CAD build for the part. Positions are in the model's coordinates, mm. A direction names the side the tool comes from. Coordinates: 2 decimals unless noted, no trailing zeros. Order: outer loops, then holes, each group sorted by start corner. A loop starts at its lowest first (then second) coordinate and runs counter-clockwise, first axis right, second up. Notation, with made-up numbers: (54, 72.5) - (77, 72.5) arc R23 cw to (77, 83.5) - close; hole circle Ø2 at (-8, 53). An arc over 180 degrees is marked (long way). Use one line per item in the form item = value.
```python
from build123d import *
from OCP.BRepFilletAPI import BRepFilletAPI_MakeChamfer

# Parameters (mm, degrees)
SKETCH_1_W          = 220
SKETCH_1_H          = 70
SKETCH_1_R          = 2.1
SKETCH_1_R_2        = 11
EXTRUDE_1_DEPTH     = 3
SKETCH_2_R          = 4
CUT_EXTRUDE_1_DEPTH = 116.589791937
CUT_EXTRUDE_2_DEPTH = 116.589791937
CHAMFER_1_SIZE      = 2
CUT_EXTRUDE_3_DEPTH = 116.589791937
CHAMFER_3_SIZE      = 4
CHAMFER_3_SIZE2     = 5.201672953


with BuildPart() as part:
    # 草图1 → 凸台-拉伸1 (new, symmetric)
    with BuildSketch(Plane(origin=(0, 0, 0), x_dir=(1, 0, 0), z_dir=(0, 1, 0))):
        Rectangle(SKETCH_1_W, SKETCH_1_H)
        with Locations(Location((-100, 25, 0), (0, 0, 270))):
            Circle(SKETCH_1_R, mode=Mode.SUBTRACT)
        with Locations(Location((100, 25, 0), (0, 0, 270))):
            Circle(SKETCH_1_R, mode=Mode.SUBTRACT)
        with Locations(Location((0, 29, 0), (0, 0, 270))):
            Circle(SKETCH_1_R, mode=Mode.SUBTRACT)
        with Locations(Location((25.11473671, -14.5, 0), (0, 0, 270))):
            Circle(SKETCH_1_R, mode=Mode.SUBTRACT)
        with Locations(Location((-25.11473671, -14.5, 0), (0, 0, 270))):
            Circle(SKETCH_1_R, mode=Mode.SUBTRACT)
        with Locations(Location((0, 0, 0), (0, 0, 270))):
            Circle(SKETCH_1_R_2, mode=Mode.SUBTRACT)
        with Locations(Location((-100, -9, 0), (0, 0, 270))):
            Circle(SKETCH_1_R, mode=Mode.SUBTRACT)
        with Locations(Location((100, -9, 0), (0, 0, 270))):
            Circle(SKETCH_1_R, mode=Mode.SUBTRACT)
    extrude(amount=EXTRUDE_1_DEPTH, both=True)

    # 草图2 → 切除-拉伸1 (cut, through all)
    with BuildSketch(Plane(origin=(0, 3, 0), x_dir=(1, 0, 0), z_dir=(0, 1, 0))):
        with Locations(Location((16.670989023, -9.625, 0), (0, 0, 270))):
            Circle(SKETCH_2_R)
    extrude(amount=-CUT_EXTRUDE_1_DEPTH, mode=Mode.SUBTRACT)

    # 草图3 → 切除-拉伸2 (cut, through all)
    with BuildSketch(Plane(origin=(0, 3, 0), x_dir=(1, 0, 0), z_dir=(0, 1, 0))):
        with BuildLine():
            Line((4.6, -20.3), (4.6, -16.7))
            ThreePointArc((4.6, -16.7), (4.014213562, -15.285786438), (2.6, -14.7))
            Line((2.6, -14.7), (-2.6, -14.7))
            ThreePointArc((-2.6, -14.7), (-4.014213562, -15.285786438), (-4.6, -16.7))
            Line((-4.6, -16.7), (-4.6, -20.3))
            ThreePointArc((-4.6, -20.3), (-4.014213562, -21.714213562), (-2.6, -22.3))
            Line((-2.6, -22.3), (2.6, -22.3))
            ThreePointArc((2.6, -22.3), (4.014213562, -21.714213562), (4.6, -20.3))
        make_face()
    extrude(amount=-CUT_EXTRUDE_2_DEPTH, mode=Mode.SUBTRACT)

    # 倒角1
    chamfer_1_edges = [part.edges().sort_by_distance(p)[0] for p in [
        (0, 3, -31.1),
        (25.11473671, 3, 12.4),
        (-25.11473671, 3, 12.4),
    ]]
    chamfer(chamfer_1_edges, length=CHAMFER_1_SIZE)

    # 草图5 → 切除-拉伸3 (cut, through all)
    with BuildSketch(Plane(origin=(0, 3, 0), x_dir=(1, 0, 0), z_dir=(0, 1, 0))):
        Polygon((-110, -19), (-35.11473671, -35), (-110, -35), align=None)
        Polygon((35.11473671, -35), (110, -35), (110, -19), align=None)
    extrude(amount=-CUT_EXTRUDE_3_DEPTH, mode=Mode.SUBTRACT)

    # 倒角3: one chamfer whose edges measure the first distance from different faces: ONE call of the kernel's chamfer builder (chamfer() names one face for all edges)
    chamfer_3_edges_1 = [part.edges().sort_by_distance(p)[0] for p in [
        (110, 0, 19),
    ]]
    chamfer_3_side_1 = [part.faces().sort_by_distance(p)[0] for p in [
        (110, 0, -8),
    ]]
    chamfer_3_edges_2 = [part.edges().sort_by_distance(p)[0] for p in [
        (-110, 0, -35),
        (110, 0, -35),
    ]]
    chamfer_3_edges_3 = [part.edges().sort_by_distance(p)[0] for p in [
        (-110, 0, 19),
    ]]
    chamfer_3_side_3 = [part.faces().sort_by_distance(p)[0] for p in [
        (-110, 0, -8),
    ]]
    chamfer_3 = BRepFilletAPI_MakeChamfer(part.part.solid().wrapped)
    for e in chamfer_3_edges_1:
        chamfer_3.Add(CHAMFER_3_SIZE, CHAMFER_3_SIZE2, e.wrapped, chamfer_3_side_1[0].wrapped)  # the first distance lies on this face
    for e in chamfer_3_edges_2:
        chamfer_3.Add(CHAMFER_3_SIZE, e.wrapped)
    for e in chamfer_3_edges_3:
        chamfer_3.Add(CHAMFER_3_SIZE, CHAMFER_3_SIZE2, e.wrapped, chamfer_3_side_3[0].wrapped)  # the first distance lies on this face
    add(Compound.cast(chamfer_3.Shape()), mode=Mode.REPLACE)


solid = part.part
```
Item 1: Drill centre lines: line 1 (X direction, y = -1.05, z = 14.5); line 2 (X direction, y = -1, z = -25); line 3 (X direction, y = 1.75, z = 0.5). Where is each one in solid material? Low to high. Write a range as [from, to].
Derived:
line_1 = [-110, -27.21], [-23.01, 23.01], [27.21, 110]
line_2 = [-110, -102.1], [-97.9, 97.9], [102.1, 110]
line_3 = [-110, -10.99], [10.99, 110]
Item 2: Cut at D-D, the plane y = -1.5. State how many separate pieces and enclosed holes the cut face has, plus the area to 3 significant figures.
Derived:
separate_pieces = 1
enclosed_holes = 10
area = 13,600 mm²
Item 3: Drop flat-ended pins along their axis: pin 1 (1.8 mm diameter, centred on y = -0.5, z = 17.5, fed in from +X); pin 2 (1.1 mm diameter, centred on y = 0.5, z = 19, fed in from -X). Give the stop position or say it passes through.
Derived:
pin_1 = 108.4
pin_2 = -106.55
Item 4: Cut at A-A, the plane z = 0. Write the cut outline in (x, y), plus the area to 3 significant figures.
Derived:
outline = (-110, -3) - (-11, -3) - (-11, 3) - (-110, 3) - close; (11, -3) - (110, -3) - (110, 3) - (11, 3) - close
area = 1,190 mm²
Item 5: 3-axis set-ups, long thin cutter, end or side, ignore diameter. For faces 1 (the face through (4.6, 0, 19)), 2 (the face through (110, 0, -8)): which of +Z, -Z, +X, -X, +Y, -Y reach the whole face in a straight line?
Derived:
face_1 = +Y, -Y
face_2 = +Z, -Z, +X, +Y, -Y
Item 6: Two-plate mould, pull along X, no slides. Class faces 3 (the face through (-2, 3, -16)), 4 (the face through (108, 0, -33)), 5 (the face through (-27.165, -1.028, 14.045)): +X half, -X half, draft (parallel to the pull), parting line (faces both ways), or undercut.
Derived:
face_3 = draft
face_4 = +X half
face_5 = undercut
Item 7: Cut at B-B, the plane x = 0. Write the cut outline in (y, z), plus the area to 3 significant figures.
Derived:
outline = (-3, -35) - (3, -35) - (3, -33.1) - (1, -31.1) - (-3, -31.1) - close; (-3, -26.9) - (1, -26.9) - (3, -24.9) - (3, -11) - (-3, -11) - close; (-3, 11) - (3, 11) - (3, 14.7) - (-3, 14.7) - close; (-3, 22.3) - (3, 22.3) - (3, 35) - (-3, 35) - close
area = 213 mm²
Item 8: Cut at C-C, the plane x = 100. Write the cut outline in (y, z).
Derived:
outline = (-3, -35) - (3, -35) - (3, -27.1) - (-3, -27.1) - close; (-3, -22.9) - (3, -22.9) - (3, 6.9) - (-3, 6.9) - close; (-3, 11.1) - (3, 11.1) - (3, 21.14) - (-3, 21.14) - close
